```python
from build123d import *

# Parameters (mm, degrees)
SKETCH_1_W          = 129.003888627
SKETCH_1_H          = 71.620980981
SKETCH_1_R          = 1.6
EXTRUDE_1_DEPTH     = 3
SKETCH_2_R          = 2.65
CUT_EXTRUDE_1_DEPTH = 3
SKETCH_3_R          = 2.65
CUT_EXTRUDE_2_DEPTH = 3


with BuildPart() as part:
    # 草图1 → 凸台-拉伸1 (new body)
    with BuildSketch(Plane.XY):
        with Locations((-64.501944314, -11.78950951)):
            Rectangle(SKETCH_1_W, SKETCH_1_H)
        with Locations((-14, -29.6)):
            Circle(SKETCH_1_R, mode=Mode.SUBTRACT)
        with Locations((-14, -41.6)):
            Circle(SKETCH_1_R, mode=Mode.SUBTRACT)
        with Locations((-14, 6)):
            Circle(SKETCH_1_R, mode=Mode.SUBTRACT)
        with Locations((-14, 18)):
            Circle(SKETCH_1_R, mode=Mode.SUBTRACT)
        with Locations((-90.004518872, 18.016885816)):
            Circle(SKETCH_1_R, mode=Mode.SUBTRACT)
        with Locations((-90.005778933, 6.016885882)):
            Circle(SKETCH_1_R, mode=Mode.SUBTRACT)
        with Locations((-90.010777175, -41.583113855)):
            Circle(SKETCH_1_R, mode=Mode.SUBTRACT)
        with Locations((-90.009517114, -29.583113922)):
            Circle(SKETCH_1_R, mode=Mode.SUBTRACT)
        with Locations((-115.010777037, -41.580488728)):
            Circle(SKETCH_1_R, mode=Mode.SUBTRACT)
        with Locations((-115.009516976, -29.580488794)):
            Circle(SKETCH_1_R, mode=Mode.SUBTRACT)
        with Locations((-115.005778795, 6.019511009)):
            Circle(SKETCH_1_R, mode=Mode.SUBTRACT)
        with Locations((-115.004518734, 18.019510943)):
            Circle(SKETCH_1_R, mode=Mode.SUBTRACT)
    extrude(amount=EXTRUDE_1_DEPTH)

    # 草图2 → 切除-拉伸1 (cut)
    with BuildSketch(Plane.XY.offset(3)):
        with Locations((-58.1, -11.789509509)):
            Circle(SKETCH_2_R)
    extrude(amount=-CUT_EXTRUDE_1_DEPTH, mode=Mode.SUBTRACT)

    # 草图3 → 切除-拉伸2 (cut)
    with BuildSketch(Plane.XY.offset(3)):
        with Locations((-80.6, -11.789509509)):
            Circle(SKETCH_3_R)
        with Locations((-35.6, -11.789509509)):
            Circle(SKETCH_3_R)
    extrude(amount=-CUT_EXTRUDE_2_DEPTH, mode=Mode.SUBTRACT)


solid = part.part
```
Check sheet for the modelled part. Datum: model origin and axes. Units: mm. Round coordinates to 2 decimals unless told otherwise and drop trailing zeros. Answer as a JSON object with one key per item and string values. Group by question number.
Q1. Mould release check, pull along Y, two halves, no side actions. Record for faces 1 (the face through (-65, -47.6, 1)), 2 (the face through (-116.604, 6.09, 1.479)), 3 (the face through (-65, -11, 3)): released by +Y, released by -Y, zero draft, split by the parting line, or undercut.
Q2. Sectioned sample at A-A, the plane z = 1.8. Count the separate pieces of the cut face and the enclosed holes in it, plus the area to 3 significant figures.
Q3. Scan lines: line 1 along Y through (x, z) = (-14, 0.9); line 2 along X through (y, z) = (-30, 2.45); line 3 along Y through (x, z) = (-90.5, 1.9). Record each from-to range of solid material in increasing order. Write a range as [from, to].
Q4. Gauge pin test, flat end, axial feed: P1, Ø3.5, axis at x = -14, y = 6, coming from the +Z side. Record the tip position at first contact, or that the pin passes through.
Solution:
{
 "1": {"face 1": "released by -Y", "face 2": "undercut", "face 3": "zero draft"},
 "2": {"separate pieces": "1", "enclosed holes": "15", "area": "9,080 mm²"},
 "3": {"line 1": "y = [-47.6, -43.2], [-40, -31.2], [-28, 4.4], [7.6, 16.4], [19.6, 24.02]", "line 2": "x = [-129, -116.55], [-113.47, -91.55], [-88.46, -15.55], [-12.45, 0]", "line 3": "y = [-47.6, -43.11], [-40.06, -31.11], [-28.06, 4.5], [7.54, 16.5], [19.54, 24.02]"},
 "4": {"P1": "stops at z = 3"}
}
